Design review of the part built by this model. Coordinates are the model's own, in mm. A direction names the side the tool comes from. Coordinates: 2 decimals unless noted, no trailing zeros. Loops run counter-clockwise (first coordinate to the right, second up) from the corner with the lowest first, then second, coordinate; pieces in that order, holes last. Notation, with made-up numbers: (54, -35.5) -> (111, -35.5) arc R35 ccw to (111, 0.5) -> close; hole circle Ø11 at (-25, -38). An arc over 180 degrees is marked (long way). Use CSV: the item, a comma, the result in double quotes.
```python
from build123d import *

# Parameters (mm, degrees)
SKETCH_1_W          = 12
SKETCH_1_H          = 12
EXTRUDE_1_DEPTH     = 20
SKETCH_2_W          = 28
SKETCH_2_H          = 12
EXTRUDE_2_DEPTH     = 12
SKETCH_3_R          = 2.5
CUT_EXTRUDE_1_DEPTH = 20
SKETCH_4_R          = 1
CUT_EXTRUDE_2_DEPTH = 13
SKETCH_5_R          = 2
CUT_EXTRUDE_3_DEPTH = 29


with BuildPart() as part:
    # Эскиз1 → Бобышка-Вытянуть1 (new body)
    with BuildSketch(Plane(origin=(0, 0, 0), x_dir=(1, 0, 0), z_dir=(0, 1, 0))):
        Rectangle(SKETCH_1_W, SKETCH_1_H)
    extrude(amount=EXTRUDE_1_DEPTH)

    # Эскиз2 → Бобышка-Вытянуть2 (add)
    with BuildSketch(Plane(origin=(0, 20, 0), x_dir=(1, 0, 0), z_dir=(0, 1, 0))):
        Rectangle(SKETCH_2_W, SKETCH_2_H)
    extrude(amount=EXTRUDE_2_DEPTH)

    # Эскиз3 → Вырез-Вытянуть1 (cut)
    with BuildSketch(Plane.XZ):
        Circle(SKETCH_3_R)
    extrude(amount=-CUT_EXTRUDE_1_DEPTH, mode=Mode.SUBTRACT)

    # Эскиз4 → Вырез-Вытянуть2 (cut, through all)
    with BuildSketch(Plane.XY.offset(6)):
        with Locations((0, 14)):
            Circle(SKETCH_4_R)
    extrude(amount=-CUT_EXTRUDE_2_DEPTH, mode=Mode.SUBTRACT)

    # Эскиз5 → Вырез-Вытянуть3 (cut, through all)
    with BuildSketch(Plane.ZY.offset(14)):
        with Locations((0, 26)):
            Circle(SKETCH_5_R)
    extrude(amount=-CUT_EXTRUDE_3_DEPTH, mode=Mode.SUBTRACT)


solid = part.part
```
Item 1: Machinability: for faces 1 (the face through (2.385, 9.86, 0.751)), 2 (the face through (-14, 26, 3)), 3 (the face through (6, 10, 0)), 4 (the face through (-6, 10, 0)), 5 (the face through (3, 0, 0)), which of the approach directions +Z, -Z, +X, -X, +Y, -Y give a long, thin tool a straight path to every point of the face, cutting with its end or side? Answer none if there is none.
Checked values:
face 1,"-Y"
face 2,"+Z, -Z, -X, +Y, -Y"
face 3,"+Z, -Z, +X, -Y"
face 4,"+Z, -Z, -X, -Y"
face 5,"+Z, -Z, +X, -X, -Y"
Item 2: Add section A-A (x = 0). Give the boundary of the cut face in (y, z).
Checked values:
outline,"(0, -6) -> (13, -6) -> (13, -2.5) -> (0, -2.5) -> close; (0, 2.5) -> (13, 2.5) -> (13, 6) -> (0, 6) -> close; (15, -6) -> (32, -6) -> (32, 6) -> (15, 6) -> (15, 2.5) -> (20, 2.5) -> (20, -2.5) -> (15, -2.5) -> close; hole circle Ø4 at (26, 0)"
Item 3: To check wall thickness, follow line 1 along Y through (x, z) = (1.75, 0); line 2 along Z through (x, y) = (1.5, 10.5); line 3 along Y through (x, z) = (0, 3.2). State the ranges of each line that lie inside material, in increasing order.
Checked values:
line 1,"20 to 24, 28 to 32"
line 2,"-6 to -2, 2 to 6"
line 3,"0 to 13, 15 to 32"
Item 4: Clearance check with flat-ended pins moving along their axes: pin 1 (3 mm diameter, centred on x = 0, z = 0, fed in from -Y); pin 2 (2 mm diameter, centred on x = -3, z = 3, fed in from -Y); pin 3 (6 mm diameter, centred on y = 13.5, z = 1.5, fed in from -X); pin 4 (6 mm diameter, centred on y = 10, z = -2.5, fed in from +X). State where each tip first meets the part, or that it passes through.
Checked values:
pin 1,"y = 20"
pin 2,"y = 0"
pin 3,"x = -6"
pin 4,"x = 6"
Item 5: Draft analysis for pull direction Y (two halves, no side actions). For faces 6 (the face through (0, 19, -6)), 7 (the face through (-10, 20, 0)), 8 (the face through (1, 14, -4)), state which applies: pulls with the +Y half, pulls with the -Y half, needs draft (parallel to the pull), parting line crosses it, or undercut.
Checked values:
face 6,"needs draft"
face 7,"pulls with the -Y half"
face 8,"undercut"
Item 6: Add section D-D (y = 15.5). Give the boundary of the cut face in (x, z).
Checked values:
outline,"(-6, -6) -> (6, -6) -> (6, 6) -> (-6, 6) -> close; hole circle Ø5 at (0, 0)"
Item 7: Add section C-C (y = 26). Give the boundary of the cut face in (x, z).
Checked values:
outline,"(-14, -6) -> (14, -6) -> (14, -2) -> (-14, -2) -> close; (-14, 2) -> (14, 2) -> (14, 6) -> (-14, 6) -> close"
Item 8: Add section B-B (z = 0). Give the boundary of the cut face in (x, y), then the cut area to 3 significant figures.
Checked values:
outline,"(-14, 20) -> (-6, 20) -> (-6, 0) -> (-2.5, 0) -> (-2.5, 20) -> (2.5, 20) -> (2.5, 0) -> (6, 0) -> (6, 20) -> (14, 20) -> (14, 24) -> (-14, 24) -> close; (-14, 28) -> (14, 28) -> (14, 32) -> (-14, 32) -> close"
area,"364 mm^2"
